Check sheet for the modelled part. Datum: model origin and axes. Units: mm. A direction names the side the tool comes from. Give positions to 0.01 mm unless a question says otherwise; leave off trailing zeros. Order: outer loops, then holes, each group sorted by start corner. A loop starts at its lowest first (then second) coordinate and runs counter-clockwise, first axis right, second up. Notation, with made-up numbers: M 24,79.25 L 30,79.25 A21 ccw 30,106.25 Z; hole C -18,46 d7. An arc over 180 degrees is marked long. Return JSON: item names as keys, results as strings. Group by question number.
from build123d import *

# Parameters (mm, degrees)
SKETCH_1_W      = 40
SKETCH_1_H      = 22.6
EXTRUDE_1_DEPTH = 1.2
CHAMFER_1_SIZE  = 5
CHAMFER_2_SIZE  = 1


with BuildPart() as part:
    # 스케치1 → 보스-돌출1 (new, symmetric)
    with BuildSketch(Plane.XY):
        Rectangle(SKETCH_1_W, SKETCH_1_H)
        with BuildLine():
            Line((-12.5, 2.864624259), (12.5, 2.864624259))
            ThreePointArc((12.5, 2.864624259), (15.364624259, 0), (12.5, -2.864624259))
            Line((12.5, -2.864624259), (-12.5, -2.864624259))
            ThreePointArc((-12.5, -2.864624259), (-15.364624259, 0), (-12.5, 2.864624259))
        make_face(mode=Mode.SUBTRACT)
    extrude(amount=EXTRUDE_1_DEPTH, both=True)

    # 모따기1
    chamfer_1_edges = [part.edges().sort_by_distance(p)[0] for p in [
        (20, -11.3, 0),
        (-20, -11.3, 0),
        (-20, 11.3, 0),
        (20, 11.3, 0),
    ]]
    chamfer(chamfer_1_edges, length=CHAMFER_1_SIZE)

    # 모따기2
    chamfer_2_edges = [part.edges().sort_by_distance(p)[0] for p in [
        (0, 11.3, 1.2),
        (20, 0, 1.2),
        (-20, 0, 1.2),
        (0, -11.3, 1.2),
    ]]
    chamfer(chamfer_2_edges, length=CHAMFER_2_SIZE)


solid = part.part
1) Material ranges on line 1 along Y through (x, z) = (12, 0.1); line 2 along Y through (x, z) = (7, 1); line 3 along X through (y, z) = (-1, 0.9), recorded low to high.
2) Release check for a two-part mould opening along Y. For faces 1 (the face through (0, -4, 1.2)), 2 (the face through (-0.2, 10.8, 0.7)), 3 (the face through (0, -2.865, 0)) record: released by +Y, released by -Y, zero draft, split by the parting line, or undercut.
3) Sectioned sample at C-C on z = -0.75. Record the boundary of the cut face in (x, y), then the cut area to 3 significant figures.
4) Tool access check on faces 4 (the face through (-15.364, -0.063, 0.017)), 5 (the face through (20, 0, 0)). Record the directions out of +Z, -Z, +X, -X, +Y, -Y that give a thin tool (end or side, any length) a straight path to the whole face; none if there is none.
5) Sectioned sample at A-A on y = 0. Record the boundary of the cut face in (x, z).
6) Sectioned sample at D-D on x = 17. Record the boundary of the cut face in (y, z), then the cut area to 3 significant figures.
7) Sectioned sample at B-B on x = -11. Record the boundary of the cut face in (y, z).
Reply:
{
 "1": {"line 1": "-11.3 to -2.86, 2.86 to 11.3", "line 2": "-10.5 to -2.86, 2.86 to 10.5", "line 3": "-19.3 to -15.18, 15.18 to 19.3"},
 "2": {"face 1": "zero draft", "face 2": "released by +Y", "face 3": "undercut"},
 "3": {"outline": "M -20,-6.3 L -15,-11.3 L 15,-11.3 L 20,-6.3 L 20,6.3 L 15,11.3 L -15,11.3 L -20,6.3 Z; hole M -12.5,-2.86 L 12.5,-2.86 A2.86 ccw 12.5,2.86 L -12.5,2.86 A2.86 ccw Z", "area": "685 mm^2"},
 "4": {"face 4": "+Z, -Z", "face 5": "+Z, -Z, +X, +Y, -Y"},
 "5": {"outline": "M -20,-1.2 L -15.36,-1.2 L -15.36,1.2 L -19,1.2 L -20,0.2 Z; M 15.36,-1.2 L 20,-1.2 L 20,0.2 L 19,1.2 L 15.36,1.2 Z"},
 "6": {"outline": "M -9.3,-1.2 L 9.3,-1.2 L 9.3,1.2 L -9.3,1.2 Z", "area": "44.6 mm^2"},
 "7": {"outline": "M -11.3,-1.2 L -2.86,-1.2 L -2.86,1.2 L -10.3,1.2 L -11.3,0.2 Z; M 2.86,-1.2 L 11.3,-1.2 L 11.3,0.2 L 10.3,1.2 L 2.86,1.2 Z"}
}
